Build history of the part. All positions in model axes, mm. Round coordinates to 2 decimals unless told otherwise and drop trailing zeros. Loops run counter-clockwise (first coordinate to the right, second up) from the corner with the lowest first, then second, coordinate; pieces in that order, holes last. Notation, with made-up numbers: (47.25, 20.5) -> (82.25, 20.5) arc R19 ccw to (82.25, 29.5) -> close; hole circle Ø11 at (57.25, 78). An arc over 180 degrees is marked (long way). Put each result on its own line as item: value. Start each with the question number.
Item 1: Flat gauge pins, fed straight in: pin 1 Ø8 at (y, z) = (85.5, 5.5) entering from -X; pin 2 Ø6 at (x, y) = (5, 44.5) entering from -Z; pin 3 Ø10 at (x, y) = (-5.5, 125.5) entering from +Z. Where does each tip first touch, or does it go through?
Item 2: Drill centre lines: probe 1 along X at (y, z) = (132.5, -3); probe 2 along Z at (x, y) = (-3, 121); probe 3 along Z at (x, y) = (3.5, 31). Where is each one in solid material? Low to high. Write a range as [from, to].
Item 3: Cut at A-A, the plane y = 83. List the corners of the cut face in (x, z).
Autodesk Inventor part; units mm, degrees
ref_plane "Work Plane1" through (10, 0, 0) normal (1, 0, 0) x (0, 1, 0)
ref_plane "XZ Plane" through (0, 0, 0) normal (0, 1, 0) x (-1, 0, 0)
ref_plane "XY Plane" through (0, 0, 0) normal (0, 0, 1) x (1, 0, 0)
sketch "Sketch1" plane through (0, 0, 0) normal (0, 1, 0) x (-1, 0, 0)
  circle A0 centre (0, 0) radius 10
  dimension "d0" = 20
extrude "Extrusion1" add sketch "Sketch1" along normal blind 220
ref_plane "Work Plane1" through (10, 0, 0) normal (1, 0, 0) x (0, 1, 0)
sketch "Sketch2" plane through (10, 0, 0) normal (1, 0, 0) x (0, 1, 0)
  line L0 (220, -10) -> (220, 10)
  line L1 (0, -10) -> (0, 10)
  line L2 (0, 0) -> (132.5, 0)
  circle A0 centre (132.5, 0) radius 1.25
  circle A1 centre (132.5, 0) radius 0.5
  circle A2 centre (132.5, 0.0309) radius 2.5
  line L3 (0, -10) -> (0, 10)
  line L4 (132.5, -2.4691) -> (0, -2.4691)
  line L5 (0, -2.4691) -> (0, 2.5309)
  line L6 (0, 2.5309) -> (132.5, 2.5309)
  line L7 (132.5, 2.5309) -> (132.5, -2.4691)
  line L8 (220, -10) -> (220, 10)
  line L9 (132.5, -2.4691) -> (220, -2.4691)
  line L10 (220, -2.4691) -> (220, 2.5309)
  line L11 (220, 2.5309) -> (132.5, 2.5309)
  line L12 (132.5, 2.5309) -> (132.5, -2.4691)
  dimension "d21" = 5
  dimension "d3" = 132.5
  dimension "d4" = 2.5
  dimension "d5" = 1
extrude "Extrusion2" cut sketch "Sketch2" against normal blind 0.5
sketch "Sketch3" plane through (9.5, 0, 0) normal (1, 0, 0) x (0, 0, -1)
  line L0 (2.4691, 0) -> (-2.5309, 0)
  circle A0 centre (-0.0309, 132.5) radius 0.75
  circle A1 centre (-0.0309, 132.5) radius 1.25
  line L1 (2.4691, 220) -> (2.4691, 0)
  line L2 (-2.5309, 220) -> (2.4691, 220)
  line L3 (-2.5309, 0) -> (-2.5309, 220)
  point P0 (0, 0)
  dimension "d24" = 1.5
  dimension "d25" = 2.5
extrude "Extrusion4" [suppressed]
chamfer "Chamfer5" [suppressed]
chamfer "Chamfer6" distance 0.5 angle 45 2 edges at (-9.9999, 220, -0.0319) (-9.9999, 0, -0.0319)
sketch "Sketch4" plane through (9.5, 0.3156, -2.4691) normal (0, 0, 1) x (1, 0, 0)
  spline S0 degree 2 poles (0.1904, 0.1843) (0.0943, 0.0912) (0, -0.0001) knots 0 0 0 1 1 1 weights 1 1.000046 1
  line L0 (0.1904, 219.1844) -> (0.1904, 0.1844)
  spline S1 degree 4 poles (0, 219.3688) (0.0476, 219.3228) (0.0952, 219.2767) (0.1428, 219.2306) (0.1904, 219.1845) knots 0 0 0 0 0 1 1 1 1 1
  line L1 (0, 219.3687) -> (0, 0)
  point P0 (-9.5, -0.3156)
extrude "Extrusion5" cut sketch "Sketch4" against normal blind 10
sketch "Sketch5" plane through (9.5, 0.3313, 2.5309) normal (0, 0, -1) x (-1, 0, 0)
  spline S0 degree 2 poles (0, -0.0001) (-0.0865, 0.0835) (-0.1744, 0.1686) knots 0 0 0 1 1 1 weights 1 1.000039 1
  line L0 (0, 0) -> (0, 219.3373)
  spline S1 degree 2 poles (-0.1744, 219.1688) (-0.0865, 219.2539) (0, 219.3374) knots 0 0 0 1 1 1 weights 1 1.000039 1
  line L1 (-0.1744, 0.1687) -> (-0.1744, 219.1687)
  point P0 (9.5, -0.3313)
extrude "Extrusion6" cut sketch "Sketch5" against normal blind 10
properties part number "wał_półkola" material "Stainless Steel"
Reply:
1. pin 1: stops at x = -9.89
1. pin 2: stops at z = -9.8
1. pin 3: stops at z = 9.99
2. probe 1: x = [-9.54, 9.5]
2. probe 2: z = [-9.54, 9.54]
2. probe 3: z = [-9.37, 9.37]
3. outline: (9.5, -3.12) -> (9.5, 3.12) arc R10 ccw (long way) to start
